Input: part model. Units: mm. Frame: model coordinates. A direction names the side the tool comes from. Coordinates: 2 decimals unless noted, no trailing zeros. Loops run counter-clockwise (first coordinate to the right, second up) from the corner with the lowest first, then second, coordinate; pieces in that order, holes last.
(1) Section D-D, the plane y = 29. Return loops of the section in (x, z), then the cut area to 3 significant figures.
(2) Section C-C, the plane z = -11.5. Return loops of the section in (x, y).
(3) Line query: L1, parallel to Z at x = -10, y = 3.5; L2, parallel to Z at x = -62, y = 37; L3, parallel to X at y = 38.15, z = -8. Output: solid intervals per line, ascending.
(4) Contact query for flat-ended pins moving along their axis: P1, Ø2.5, axis at y = 1, z = 4.5, coming from the -X side; P2, Ø20, axis at x = -47, y = 14.5, coming from the +Z side; P3, Ø4.5, axis at x = 4, z = 18.5, coming from the +Y side; P4, Ø3, axis at x = 10, z = -17.5, coming from the -Y side. Output: stop coordinate, or through.
(5) Set-up query: faces 1 (the face through (-22, 3.3, 0)), 2 (the face through (8.82, 2.46, 16.42)), 3 (the face through (-43, 3.3, -12)). Return all of +Z, -Z, +X, -X, +Y, -Y with unobstructed straight access to the full face (end or side cutting, diameter ignored); none if empty.
(6) Section B-B, the plane x = -42. Return loops of the section in (y, z).
(7) Mould query, pull axis Y, two halves, no side actions, for faces 4 (the face through (-57, 35, 0)), 5 (the face through (15, 2, 0)), 6 (the face through (-37, 8.3, 0)), 7 (the face through (-3, 0, 0)). Classes: released by +Y, released by -Y, zero draft, split by the parting line, or undercut.
(8) Section A-A, the plane z = 8. Return loops of the section in (x, y).
```python
from build123d import *

# Parameters (mm, degrees)
SKETCH1_W                = 30
SKETCH1_H                = 45
SKETCH1_R                = 1.6
BOSS_EXTRUDE3_DEPTH      = 5
SKETCH2_W                = 64
SKETCH2_H                = 27.1
SKETCH2_W_2              = 30
BOSS_EXTRUDE4_DEPTH      = 35
BOSS_EXTRUDE4_DEPTH_BACK = 1.7
SKETCH3_W                = 4
SKETCH3_H                = 24.6
SKETCH3_W_2              = 5
SKETCH3_H_2              = 27.1
SKETCH3_W_3              = 2
BOSS_EXTRUDE5_DEPTH      = 3.3
SKETCH4_R                = 1.4
CUT_EXTRUDE1_DEPTH       = 41
CUT_EXTRUDE4_DEPTH       = 37.05
CUT_EXTRUDE5_DEPTH       = 10
CUT_EXTRUDE5_DEPTH_BACK  = 10
CUT_EXTRUDE6_DEPTH       = 37.05


with BuildPart() as part:
    # Sketch1 → Boss-Extrude3 (new body)
    with BuildSketch(Plane(origin=(0, 0, 0), x_dir=(1, 0, 0), z_dir=(0, 1, 0))):
        Rectangle(SKETCH1_W, SKETCH1_H)
        with Locations((-10, -17.5)):
            Circle(SKETCH1_R, mode=Mode.SUBTRACT)
        with Locations((10, -17.5)):
            Circle(SKETCH1_R, mode=Mode.SUBTRACT)
        with Locations((10, 17.5)):
            Circle(SKETCH1_R, mode=Mode.SUBTRACT)
        with Locations((-10, 17.5)):
            Circle(SKETCH1_R, mode=Mode.SUBTRACT)
        Polygon((-6, 22.5), (-15, 22.5), (-15, -22.5), (15, -22.5), (15, 22.5), (6, 22.5), align=None)
        with Locations((-10, -17.5)):
            Circle(SKETCH1_R, mode=Mode.SUBTRACT)
        with Locations((10, -17.5)):
            Circle(SKETCH1_R, mode=Mode.SUBTRACT)
        with Locations((-10, 17.5)):
            Circle(SKETCH1_R, mode=Mode.SUBTRACT)
        with Locations((10, 17.5)):
            Circle(SKETCH1_R, mode=Mode.SUBTRACT)
    extrude(amount=BOSS_EXTRUDE3_DEPTH)

    # Sketch2 → Boss-Extrude4 (add, two sides)
    with BuildSketch(Plane(origin=(0, 5, 0), x_dir=(1, 0, 0), z_dir=(0, 1, 0))) as boss_extrude4_sk:
        with Locations((-47, 0)):
            Rectangle(SKETCH2_W, SKETCH2_H)
        Rectangle(SKETCH2_W_2, SKETCH2_H)
    extrude(amount=BOSS_EXTRUDE4_DEPTH)
    extrude(boss_extrude4_sk.sketch, amount=-BOSS_EXTRUDE4_DEPTH_BACK)

    # Sketch3 → Boss-Extrude5 (add)
    with BuildSketch(Plane.XZ.offset(-3.3)):
        with Locations((-38, -1.25)):
            Rectangle(SKETCH3_W, SKETCH3_H)
        with Locations((-17.5, 0)):
            Rectangle(SKETCH3_W_2, SKETCH3_H_2)
        with Locations((-24, 0)):
            Rectangle(SKETCH3_W_3, SKETCH3_H_2)
    extrude(amount=BOSS_EXTRUDE5_DEPTH)

    # Sketch4 → Cut-Extrude1 (cut, through all)
    with BuildSketch(Plane(origin=(0, 40, 0), x_dir=(1, 0, 0), z_dir=(0, 1, 0))):
        with Locations((-62, 8)):
            Circle(SKETCH4_R)
        with Locations((-42, 8)):
            Circle(SKETCH4_R)
        with Locations((-42, -8)):
            Circle(SKETCH4_R)
        with Locations((-62, -8)):
            Circle(SKETCH4_R)
    extrude(amount=-CUT_EXTRUDE1_DEPTH, mode=Mode.SUBTRACT)

    # Sketch7 → Cut-Extrude4 (cut, through all)
    with BuildSketch(Plane.XY.offset(13.55)):
        Polygon((-45, 3.3), (-79, 35), (-79, 3.3), align=None)
    extrude(amount=-CUT_EXTRUDE4_DEPTH, mode=Mode.SUBTRACT)

    # Sketch8 → Cut-Extrude5 (cut, two sides)
    with BuildSketch(Plane(origin=(0, 0, 0), x_dir=(-1, 0, 0), z_dir=(0, 0, -1))) as cut_extrude5_sk:
        Polygon((79, 35), (34, 35), (34, 8.3), (40, 8.3), (40, 3.3), (51.306520611, 3.3), (51.306520611, 8.3), (79, 8.3), align=None)
    extrude(amount=CUT_EXTRUDE5_DEPTH, mode=Mode.SUBTRACT)
    extrude(cut_extrude5_sk.sketch, amount=-CUT_EXTRUDE5_DEPTH_BACK, mode=Mode.SUBTRACT)

    # Sketch9 → Cut-Extrude6 (cut, through all)
    with BuildSketch(Plane(origin=(0, 0, -13.55), x_dir=(-1, 0, 0), z_dir=(0, 0, -1))):
        Polygon((-15, 40), (-15, 5), (22.532904851, 40), align=None)
    extrude(amount=-CUT_EXTRUDE6_DEPTH, mode=Mode.SUBTRACT)


solid = part.part
```
Report:
1. outline: (-72.56, -13.55) - (-10.74, -13.55) - (-10.74, 13.55) - (-72.56, 13.55) - (-72.56, 10) - (-34, 10) - (-34, -10) - (-72.56, -10) - close
1. area: 904 mm2
2. outline: (-79, 35) - (-45, 3.3) - (-40, 3.3) - (-40, 0) - (-36, 0) - (-36, 3.3) - (-25, 3.3) - (-25, 0) - (-23, 0) - (-23, 3.3) - (-20, 3.3) - (-20, 0) - (15, 0) - (15, 5) - (-22.53, 40) - (-79, 40) - close
3. L1: z = -22.5 to -19.1, -15.9 to 15.9, 19.1 to 22.5
3. L2: z = -13.55 to -9.4, -6.6 to 6.6, 9.4 to 13.55
3. L3: x = -79 to -63.4, -60.6 to -43.4, -40.6 to -20.55
4. P1: stops at x = -40
4. P2: stops at z = 13.55
4. P3: stops at y = 5
4. P4: passes through
5. face 1: +Z, -Z, -Y
5. face 2: +Y, -Y
5. face 3: +Z, -Z, -X, -Y
6. outline: (3.3, -13.55) - (40, -13.55) - (40, -9.4) - (35, -9.4) - (35, -10) - (3.3, -10) - close; (3.3, 10) - (35, 10) - (35, 9.4) - (40, 9.4) - (40, 13.55) - (3.3, 13.55) - close; (35, -6.6) - (40, -6.6) - (40, 6.6) - (35, 6.6) - close
7. face 4: undercut
7. face 5: zero draft
7. face 6: undercut
7. face 7: released by -Y
8. outline: (-79, 35) - (-63.4, 35) - (-63.4, 40) - (-79, 40) - close; (-60.6, 35) - (-43.4, 35) - (-43.4, 40) - (-60.6, 40) - close; (-40.6, 35) - (-34, 35) - (-34, 8.3) - (-40, 8.3) - (-40, 0) - (-36, 0) - (-36, 3.3) - (-25, 3.3) - (-25, 0) - (-23, 0) - (-23, 3.3) - (-20, 3.3) - (-20, 0) - (15, 0) - (15, 5) - (-22.53, 40) - (-40.6, 40) - close
